```python
from build123d import *

# Parameters (mm, degrees)
SKETCH_1_R               = 20
EXTRUDE_1_DEPTH          = 0.0001
SKETCH_2_R               = 4.35
EXTRUDE_2_DEPTH          = 1
SKETCH_3_R               = 3.85
EXTRUDE_3_DEPTH          = 5.5
SKETCH_7_R               = 28.3
EXTRUDE_4_DEPTH          = 10
PATTERN_CIRCULAR_2_COUNT = 8
SKETCH_20_R              = 4
SKETCH_20_R_2            = 3.5
EXTRUDE_5_DEPTH          = 2
SKETCH_21_R              = 3.2
CUT_EXTRUDE_1_DEPTH      = 42.252660699
SKETCH_22_R              = 15
CUT_EXTRUDE_2_DEPTH      = 4
SKETCH_23_R              = 5.1
CUT_EXTRUDE_3_DEPTH      = 3.05
HOLE_WIZARD_M2_1_D       = 2.6
HOLE_WIZARD_M2_1_DEPTH   = 3
HOLE_WIZARD_M2_1_TIP     = 0.781118805
SKETCH_28_R              = 2.2
CUT_EXTRUDE_4_DEPTH      = 5.5


with BuildPart() as part:
    # 스케치1 → 보스-돌출1 (new body)
    with BuildSketch(Plane.XY):
        Circle(SKETCH_1_R)
    extrude(amount=EXTRUDE_1_DEPTH)

    # 스케치2 → 보스-돌출2 (add)
    with BuildSketch(Plane(origin=(0, 0, 0), x_dir=(-1, 0, 0), z_dir=(0, 0, -1))):
        with Locations(Location((0, 14.33, 0), (0, 0, 180))):
            Circle(SKETCH_2_R)
        with Locations(Location((-12.410144036, -7.165, 0), (0, 0, 180))):
            Circle(SKETCH_2_R)
        with Locations(Location((12.410144036, -7.165, 0), (0, 0, 180))):
            Circle(SKETCH_2_R)
    extrude(amount=EXTRUDE_2_DEPTH)

    # 스케치3 → 보스-돌출3 (add)
    with BuildSketch(Plane(origin=(0, 0, -1), x_dir=(-1, 0, 0), z_dir=(0, 0, -1))):
        with Locations((0, 14.33)):
            Circle(SKETCH_3_R)
        with Locations((-12.410144036, -7.165)):
            Circle(SKETCH_3_R)
        with Locations((12.410144036, -7.165)):
            Circle(SKETCH_3_R)
    extrude(amount=EXTRUDE_3_DEPTH)

    # 스케치7 → 보스-돌출4 (add)
    with BuildSketch(Plane.XY.offset(0.0001)):
        Circle(SKETCH_7_R)
    extrude(amount=EXTRUDE_4_DEPTH)

    # 스케치19 → M3 여유 구멍5 (revolve, cut)
    with BuildSketch(Plane(origin=(0, 28.3, 5.0001), x_dir=(0, 0, 1), z_dir=(1, 0, 0))):
        Polygon((0, 0), (0, 6.081549114), (1.8, 5), (1.8, 0), align=None)
    hole_wizard_m3_5 = revolve(axis=Axis((0, 34.65, 5.0001), (0, -1, 0)), mode=Mode.SUBTRACT)

    # 원형 패턴2: M3 여유 구멍5 ×8 about axis
    pattern_circular_2_axis = Axis((0, 0, 10.0001), (0, 0, 1))
    for i in range(1, PATTERN_CIRCULAR_2_COUNT):
        add(hole_wizard_m3_5.rotate(pattern_circular_2_axis, i * 360 / PATTERN_CIRCULAR_2_COUNT), mode=Mode.SUBTRACT)

    # 스케치20 → 보스-돌출5 (add)
    with BuildSketch(Plane(origin=(0, 0, 0), x_dir=(-1, 0, 0), z_dir=(0, 0, -1))):
        with Locations(Location((0, 0, 0), (0, 0, 180))):
            Circle(SKETCH_20_R)
        Circle(SKETCH_20_R_2, mode=Mode.SUBTRACT)
    extrude(amount=EXTRUDE_5_DEPTH)

    # 스케치21 → 컷-돌출1 (cut, through all)
    with BuildSketch(Plane(origin=(0, 0, 0), x_dir=(-1, 0, 0), z_dir=(0, 0, -1))):
        Circle(SKETCH_21_R)
    extrude(amount=-CUT_EXTRUDE_1_DEPTH, mode=Mode.SUBTRACT)

    # 스케치22 → 컷-돌출2 (cut)
    with BuildSketch(Plane.XY.offset(10.0001)):
        Circle(SKETCH_22_R)
    extrude(amount=-CUT_EXTRUDE_2_DEPTH, mode=Mode.SUBTRACT)

    # 스케치23 → 컷-돌출3 (cut)
    with BuildSketch(Plane.XY.offset(6.0001)):
        Circle(SKETCH_23_R)
    extrude(amount=-CUT_EXTRUDE_3_DEPTH, mode=Mode.SUBTRACT)

    # M2 여유 구멍1
    with Locations(Plane(origin=(0, 10, 6.0001), x_dir=(1, 0, 0), z_dir=(0, 0, 1))):
        with Locations((0, 0), (-8.660254038, -15), (8.660254038, -15)):
            Hole(HOLE_WIZARD_M2_1_D / 2, depth=HOLE_WIZARD_M2_1_DEPTH)
            with Locations((0, 0, -(HOLE_WIZARD_M2_1_DEPTH + HOLE_WIZARD_M2_1_TIP / 2))):  # 118° drill point
                Cone(0, HOLE_WIZARD_M2_1_D / 2, HOLE_WIZARD_M2_1_TIP, mode=Mode.SUBTRACT)

    # 스케치28 → 컷-돌출4 (cut)
    with BuildSketch(Plane(origin=(0, 0, -6.5), x_dir=(-1, 0, 0), z_dir=(0, 0, -1))):
        with Locations((0, 14.33)):
            Circle(SKETCH_28_R)
        with Locations((-12.410144036, -7.165)):
            Circle(SKETCH_28_R)
        with Locations((12.410144036, -7.165)):
            Circle(SKETCH_28_R)
    extrude(amount=-CUT_EXTRUDE_4_DEPTH, mode=Mode.SUBTRACT)


solid = part.part
```
The model under review builds one solid part; all positions refer to its coordinate system, in mm. A direction names the side the tool comes from. Round coordinates to 2 decimals unless told otherwise and drop trailing zeros. Write each loop counter-clockwise with the first axis right and the second up, starting at its lowest first coordinate (ties: lowest second). Pieces come first, ordered by that corner, then holes. Notation, with made-up numbers: (60.5, -1) - (111.5, -1) arc R17 cw to (111.5, 27) - close; hole circle Ø2 at (11, -31). An arc over 180 degrees is marked (long way). One line per question, with ' | ' between items.
Item 1: For faces 1 (the face through (2, 18, -1)), 2 (the face through (0.277, 22.406, 5.144)), 3 (the face through (-14.985, 0.66, 8.028)), list the 3-axis set-ups (+Z, -Z, +X, -X, +Y, -Y) from which the entire face can be reached by the end or side of a thin tool; tool diameter is ignored.
Resolved:
face 1: -Z | face 2: +Y | face 3: +Z
Item 2: To check wall thickness, follow probe 1 along Z at (x, y) = (0, 24.95); probe 2 along Y at (x, z) = (0, 7.4); probe 3 along X at (y, z) = (-8.5, -3.5). State the ranges of each line that lie inside material, in increasing order.
Resolved:
probe 1: z = 0 to 3.2, 6.8 to 10 | probe 2: y = -28.3 to -15, 15 to 28.3 | probe 3: x = -16.02 to -14.16, -10.66 to -8.8, 8.8 to 10.66, 14.16 to 16.02
Item 3: Add section A-A, the plane z = -4.75. Give the boundary of the cut face in (x, y) (3 decimals).
Resolved:
outline: circle Ø7.7 at (-12.41, -7.165); circle Ø7.7 at (0, 14.33); circle Ø7.7 at (12.41, -7.165); hole circle Ø4.4 at (-12.41, -7.165); hole circle Ø4.4 at (0, 14.33); hole circle Ø4.4 at (12.41, -7.165)
Item 4: For P1, Ø10, axis at x = -3, y = -6, coming from the -Z side; P2, Ø3, axis at x = 0, z = 5, coming from the +Y side; P3, Ø4, axis at y = -9.5, z = 8, coming from the +X side; P4, Ø3, axis at x = -18, z = -2.5, coming from the +Y side (1 decimal), all flat-tipped, find the tip position at first contact; note any pin that passes through.
Resolved:
P1: stops at z = -2 | P2: stops at y = 23.12 | P3: stops at x = 27.29 | P4: passes through
Item 5: The part is to be moulded in two halves that separate along Z. For faces 4 (the face through (-0.3, -4.2, 0)), 5 (the face through (-0.277, -22.406, 5.144)), 6 (the face through (0.17, 11.29, 4.48)), say which applies: pulls with the +Z half, pulls with the -Z half, needs draft (parallel to the pull), parting line crosses it, or undercut.
Resolved:
face 4: pulls with the -Z half | face 5: undercut | face 6: needs draft
Item 6: Add section D-D, the plane y = 25.5. Give the boundary of the cut face in (x, z).
Resolved:
outline: (-12.27, 0) - (12.27, 0) - (12.27, 10) - (-12.27, 10) - close; hole circle Ø3.6 at (0, 5)
